Here's the drawing with two shaded views (mm, measured from the low corner). I have some questions. Give positions to 0.01 mm unless a question says otherwise; leave off trailing zeros. Write each loop counter-clockwise with the first axis right and the second up, starting at its lowest first coordinate (ties: lowest second). Pieces come first, ordered by that corner, then holes. Notation, with made-up numbers: M 24,46.5 L 57,46.5 A16 ccw 57,74.5 Z; hole C 84.5,-11 d7. An arc over 180 degrees is marked long. Answer as a JSON object with one key per item and string values. Group by question number.
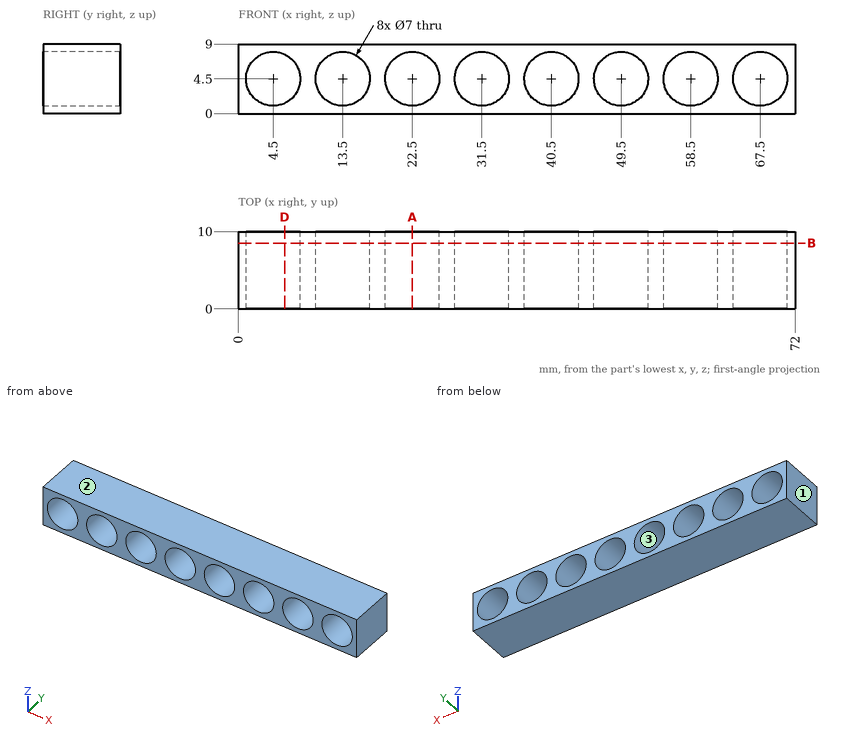
1) If we section it at A-A, the plane x = 22.5: List the corners of the cut face in (y, z) for me.
2) If we section it at D-D, the plane x = 6: List the corners of the cut face in (y, z) for me, plus the area to 3 significant figures.
3) Please list where these lines run through material, in increasing order: line 1 along Z through (x, y) = (56.5, 4.25); line 2 along Z through (x, y) = (58, 6.75). Write a range as from..to.
4) We'd pull the mould along Z, two halves only. Please class the marked faces 1, 2 and 3: released by +Z, released by -Z, zero draft, split by the parting line, or undercut.
5) If we section it at B-B, the plane y = 8.5: Give the number of separate pieces and of enclosed holes in the cut face, plus the area to 3 significant figures.
Taken from the geometry:
{
 "1": {"outline": "M 0,0 L 10,0 L 10,1 L 0,1 Z; M 0,8 L 10,8 L 10,9 L 0,9 Z"},
 "2": {"outline": "M 0,0 L 10,0 L 10,1.34 L 0,1.34 Z; M 0,7.66 L 10,7.66 L 10,9 L 0,9 Z", "area": "26.8 mm²"},
 "3": {"line 1": "0..1.63, 7.37..9", "line 2": "0..1.04, 7.96..9"},
 "4": {"face 1": "zero draft", "face 2": "released by +Z", "face 3": "undercut"},
 "5": {"separate pieces": "1", "enclosed holes": "8", "area": "340 mm²"}
}
